from build123d import *

# Parameters (mm, degrees)
SKETCH_1_R      = 15
SKETCH_1_R_2    = 10
EXTRUDE_1_DEPTH = 10
SKETCH_2_R      = 15
EXTRUDE_2_DEPTH = 40


with BuildPart() as part:
    # 草圖1 → 填料-伸長1 (new body)
    # profile 1 of 4: a face of its own
    with BuildSketch(Plane(origin=(0, 0, 0), x_dir=(1, 0, 0), z_dir=(0, 1, 0))):
        with BuildLine():
            ThreePointArc((-10, 0), (-14.393398282, -10.606601718), (-25, -15))
            Line((-25, -15), (25, -15))
            ThreePointArc((25, -15), (13.961765699, 10.156642335), (39.948186374, 1.245682198))
            Line((39.948186374, 1.245682198), (14.948186374, 301.245682198))
            ThreePointArc((14.948186374, 301.245682198), (14.987040996, 300.623379658), (15, 300))
            ThreePointArc((15, 300), (-0.623379658, 285.012959004), (-14.948186374, 301.245682198))
            Line((-14.948186374, 301.245682198), (-39.948186374, 1.245682198))
            ThreePointArc((-39.948186374, 1.245682198), (-24.376620342, 14.987040996), (-10, 0))
        make_face()
    # profile 2 of 4: a face of its own
    with BuildSketch(Plane(origin=(0, 0, 0), x_dir=(1, 0, 0), z_dir=(0, 1, 0))):
        with Locations((-25, 0)):
            Circle(SKETCH_1_R)
        with Locations(Location((-25, 0, 0), (0, 0, 270))):
            Circle(SKETCH_1_R_2, mode=Mode.SUBTRACT)
    # profile 3 of 4: a face of its own
    with BuildSketch(Plane(origin=(0, 0, 0), x_dir=(1, 0, 0), z_dir=(0, 1, 0))):
        with Locations((25, 0)):
            Circle(SKETCH_1_R)
        with Locations(Location((25, 0, 0), (0, 0, 270))):
            Circle(SKETCH_1_R_2, mode=Mode.SUBTRACT)
    # profile 4 of 4: a face of its own
    with BuildSketch(Plane(origin=(0, 0, 0), x_dir=(1, 0, 0), z_dir=(0, 1, 0))):
        with Locations((0, 300)):
            Circle(SKETCH_1_R)
        with Locations(Location((0, 300, 0), (0, 0, 270))):
            Circle(SKETCH_1_R_2, mode=Mode.SUBTRACT)
    extrude(amount=EXTRUDE_1_DEPTH)

    # 草圖2 → 填料-伸長2 (add)
    with BuildSketch(Plane(origin=(0, 10, 0), x_dir=(1, 0, 0), z_dir=(0, 1, 0))):
        with Locations(Location((0, 300, 0), (0, 0, 4.763641691))):
            Circle(SKETCH_2_R)
    extrude(amount=EXTRUDE_2_DEPTH)


solid = part.part
Input: part model. Units: mm. Frame: model coordinates. A direction names the side the tool comes from. Round coordinates to 2 decimals unless told otherwise and drop trailing zeros. Write each loop counter-clockwise with the first axis right and the second up, starting at its lowest first coordinate (ties: lowest second). Pieces come first, ordered by that corner, then holes.
1) Cut plane C-C (y = 24). Return the cut outline in (x, z), then the cut area to 3 significant figures.
2) Reachability of faces 4 (the flat face through (0, 50, -300)), 5 (the cylindrical face through (0, 5, -310)) from +Z, -Z, +X, -X, +Y, -Y: full face, straight path, thin tool, end or side. Return the list, or none.
3) Cut plane A-A (x = 19). Return the cut outline in (y, z), then the cut area to 3 significant figures.
4) Contact query for flat-ended pins moving along their axis: P1, Ø12, axis at x = 10.5, y = 34, coming from the +Z side; P2, Ø6, axis at x = -9.5, y = 11, coming from the -Z side; P3, Ø10, axis at x = -3.5, z = -77.5, coming from the +Y side; P4, Ø22, axis at x = 2.5, z = -298, coming from the -Y side. Output: stop coordinate, or through.
5) Ray query, L1, parallel to X at y = 6, z = 0; L2, parallel to X at y = 3, z = -300; L3, parallel to Y at x = -12.5, z = -238.5. Return the intervals inside material, ascending.
6) Draft query along Z for faces 1 (the cylindrical face through (-15.085, 4.93, -1.302)), 2 (the flat face through (27.623, 4.93, -149.146)), 3 (the flat face through (-1, 0, -116)). Return one class per face: pulls with the +Z half, pulls with the -Z half, needs draft (parallel to the pull), parting line crosses it, or undercut.
7) Cut plane D-D (z = -181.5). Return the cut outline in (x, y), then the cut area to 3 significant figures.
8) Cut plane B-B (x = 0). Return the cut outline in (y, z), then the cut area to 3 significant figures.
Geometry says:
1. outline: circle Ø30 at (0, -300)
1. area: 707 mm2
2. face 4: +Z, -Z, +X, -X, +Y
2. face 5: -Y
3. outline: (0, -252.62) - (10, -252.62) - (10, -8) - (0, -8) - close; (0, 8) - (10, 8) - (10, 15) - (0, 15) - close
3. area: 2,520 mm2
4. P1: stops at z = -285.69
4. P2: stops at z = -313.52
4. P3: stops at y = 10
4. P4: stops at y = 0
5. L1: x = -40 to -35, -15 to 15, 35 to 40
5. L2: x = -15.05 to -10, 10 to 15.05
5. L3: y = 0 to 10
6. face 1: undercut
6. face 2: pulls with the -Z half
6. face 3: needs draft
7. outline: (-24.93, 0) - (24.93, 0) - (24.93, 10) - (-24.93, 10) - close
7. area: 499 mm2
8. outline: (0, -315) - (50, -315) - (50, -285) - (10, -285) - (10, 15) - (0, 15) - (0, -290) - (10, -290) - (10, -310) - (0, -310) - close
8. area: 4,300 mm2
